```python
from build123d import *

# Parameters (mm, degrees)
BOSS_EXTRUDE1_DEPTH            = 35
M3_CLEARANCE_HOLE2_D           = 3.4
CBORE_FOR_M3_SHCS1_D           = 3.4
CBORE_FOR_M3_SHCS1_CBORE_D     = 6.5
CBORE_FOR_M3_SHCS1_CBORE_DEPTH = 3
TAP_DRILL_FOR_M6X1_0_TAP1_D    = 5


with BuildPart() as part:
    # Sketch1 → Boss-Extrude1 (new body)
    with BuildSketch(Plane.XY):
        Polygon((0, 9), (-3, 9), (-3, -31), (0, -31), (5, -31), (5, -9), (0, -9), align=None)
    extrude(amount=-BOSS_EXTRUDE1_DEPTH)

    # M3 Clearance Hole2 (through all)
    with Locations(Plane.ZY.offset(3)):
        with Locations((-7.5, 0), (-27.5, 0)):
            Hole(M3_CLEARANCE_HOLE2_D / 2)

    # CBORE for M3 SHCS1 (through all)
    with Locations(Plane.ZY.offset(3)):
        with Locations((-7.5, -25), (-27.5, -25)):
            CounterBoreHole(CBORE_FOR_M3_SHCS1_D / 2, CBORE_FOR_M3_SHCS1_CBORE_D / 2, CBORE_FOR_M3_SHCS1_CBORE_DEPTH)

    # Tap Drill for M6x1.0 Tap1 (through all)
    with Locations(Plane.ZY.offset(3)):
        with Locations((-17.5, -13)):
            Hole(TAP_DRILL_FOR_M6X1_0_TAP1_D / 2)


solid = part.part
```
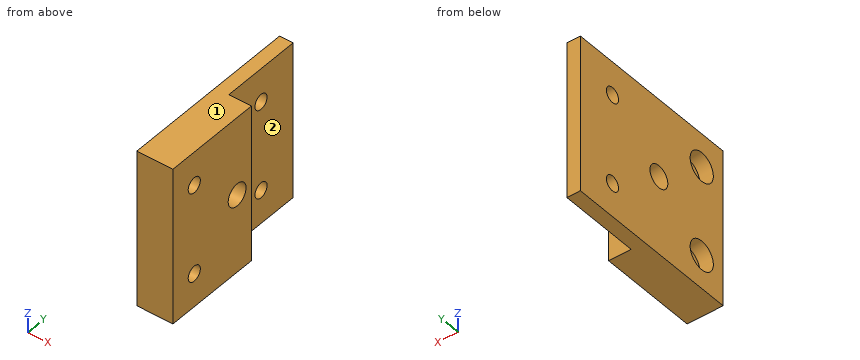
Geometry check sheet. Reference: the model listing, model coordinates, mm. Face numbers are marked on the shaded views. A direction names the side the tool comes from. Give positions to 0.01 mm unless a question says otherwise; leave off trailing zeros. Order: outer loops, then holes, each group sorted by start corner. A loop starts at its lowest first (then second) coordinate and runs counter-clockwise, first axis right, second up. Notation, with made-up numbers: (30, 54) - (57, 54) arc R16 cw to (57, 67) - close; hole circle Ø8 at (-3.5, 42). An arc over 180 degrees is marked (long way). Write item = value, one per line. Start each with the question number.
1) Section check B-B (y = 0). Enter the section's corners in (x, z).
2) Gauge pin test, flat ends, axial feed: pin 1 Ø4 at (y, z) = (-25, -27.5) entering from -X; pin 2 Ø1.5 at (x, z) = (3, -25) entering from +Y; pin 3 Ø14.5 at (y, z) = (4.5, -11.5) entering from +X. Record the tip position at first contact, or that the pin passes through.
3) Access from +Z, -Z, +X, -X, +Y, -Y to the whole of each face (thin tool, end or side, straight path). Record for the marked faces 1 and 2.
4) Section check A-A (z = -17.5). Enter the section's corners in (x, y).
5) Section check D-D (x = 1.75). Enter the section's corners in (y, z), then the cut area to 3 significant figures.
6) Section check C-C (x = -1). Enter the section's corners in (y, z), then the cut area to 3 significant figures.
7) Scan lines: L1, parallel to Y at x = 2.75, z = -27.5; L2, parallel to Y at x = 1.25, z = -17.5; L3, parallel to Y at x = 4.5, z = -10. Record each from-to range of solid material in increasing order.
Geometry check:
q1.outline = (-3, -35) - (0, -35) - (0, -29.2) - (-3, -29.2) - close; (-3, -25.8) - (0, -25.8) - (0, -9.2) - (-3, -9.2) - close; (-3, -5.8) - (0, -5.8) - (0, 0) - (-3, 0) - close
q2.pin_1 = 0
q2.pin_2 = -9
q2.pin_3 = 0
q3.face_1 = +Z, +X, -X, +Y, -Y
q3.face_2 = +Z, -Z, +X, +Y
q4.outline = (-3, -31) - (5, -31) - (5, -15.5) - (-3, -15.5) - close; (-3, -10.5) - (5, -10.5) - (5, -9) - (0, -9) - (0, 9) - (-3, 9) - close
q5.outline = (-31, -35) - (-9, -35) - (-9, 0) - (-31, 0) - close; hole circle Ø3.4 at (-25, -27.5); hole circle Ø3.4 at (-25, -7.5); hole circle Ø5 at (-13, -17.5)
q5.area = 732 mm2
q6.outline = (-31, -35) - (9, -35) - (9, 0) - (-31, 0) - close; hole circle Ø6.5 at (-25, -27.5); hole circle Ø6.5 at (-25, -7.5); hole circle Ø5 at (-13, -17.5); hole circle Ø3.4 at (0, -27.5); hole circle Ø3.4 at (0, -7.5)
q6.area = 1,300 mm2
q7.L1 = -31 to -26.7, -23.3 to -9
q7.L2 = -31 to -15.5, -10.5 to -9
q7.L3 = -31 to -9
